Here's how the part is built. I have some questions about the finished solid (model axes, mm). A direction names the side the tool comes from. Round coordinates to 2 decimals unless told otherwise and drop trailing zeros. Order: outer loops, then holes, each group sorted by start corner. A loop starts at its lowest first (then second) coordinate and runs counter-clockwise, first axis right, second up. Notation, with made-up numbers: M 15,-14 L 20,-14 A14 cw 20,-8 Z; hole C 11.5,61.5 d6. An arc over 180 degrees is marked long. Write item = value, one per line. Start each with the question number.
Item 1: I'm going to push flat-ended pins straight in: P1, Ø10, axis at x = 41, z = 9.5, coming from the -Y side; P2, Ø10, axis at x = 25, z = 19.05, coming from the -Y side. Where does each tip first touch, or does it pass through?
Item 2: I want a section at C-C, the plane z = 0. List the corners of the cut face in (x, y) for me, plus the area to 3 significant figures.
Item 3: I want a section at D-D, the plane x = 6. List the corners of the cut face in (y, z) for me.
Item 4: Please list where these lines run through material, in increasing order: L1, parallel to Z at x = 41.5, y = 3.6; L2, parallel to Z at x = 25, y = 13.75; L3, parallel to Z at x = 41.5, y = 7.
Item 5: I want a section at B-B, the plane y = 4. List the corners of the cut face in (x, z) for me.
Item 6: For faces 1 (the face through (36, 15, -11)), 2 (the face through (44, 5.994, -7)), 3 (the face through (39.985, 14.113, 0.66)), which set-ups out of +Z, -Z, +X, -X, +Y, -Y let a thin tool reach every point of the face, with its end or its side?
Item 7: We'd pull the mould along X, two halves only. Please class faces 4 (the face through (1.528, 8.458, -23.551)), 5 (the face through (48.472, 8.458, -23.551)), 6 (the face through (27.52, 10.56, 17.12)): pulls with the +X half, pulls with the -X half, needs draft (parallel to the pull), parting line crosses it, or undercut.
Item 8: I want a section at A-A, the plane x = 25. List the corners of the cut face in (y, z) for me.
```python
from build123d import *

# Parameters (mm, degrees)
F1_DEPTH       = 50
F3_D           = 6.35
F3_CBORE_D     = 10.16
F3_CBORE_DEPTH = 5.9944
F5_DEPTH       = 50.001
F6_R           = 5.08
F7_R           = 15
F7_R_2         = 13
F8_DEPTH       = 1.8


with BuildPart() as f1:
    # F0 (on Right) → F1 (new body)
    with BuildSketch(Plane.YZ):
        Polygon((0, 25), (0, 0), (0, -25), (15, -25), (15, 25), align=None)
    extrude(amount=F1_DEPTH)

    # F3 (through all)
    with Locations(Plane.XZ):
        with Locations((25, 19.052559), (8.5, 9.526279), (41.5, 9.526279), (41.5, -9.526279), (25, -19.052559), (8.5, -9.526279)):
            CounterBoreHole(F3_D / 2, F3_CBORE_D / 2, F3_CBORE_DEPTH)

    # F4 (on face) → F5 (cut, through all)
    with BuildSketch(Plane.XY.offset(25)):
        Polygon((50, 0), (50, 3), (38, 0), align=None)
        Polygon((0, 0), (12, 0), (0, 3), align=None)
    extrude(amount=-F5_DEPTH, mode=Mode.SUBTRACT)

    # F6
    f6_edges = [f1.edges().sort_by_distance(p)[0] for p in [
        (50, 9, 25),
        (0, 9, 25),
        (0, 9, -25),
        (50, 9, -25),
    ]]
    fillet(f6_edges, radius=F6_R)

    # F7 (on face) → F8 (cut)
    with BuildSketch(Plane(origin=(0, 15, 0), x_dir=(-1, 0, 0), z_dir=(0, 1, 0))):
        with Locations((-25, 0)):
            Circle(F7_R)
        with Locations((-25, 0)):
            Circle(F7_R_2, mode=Mode.SUBTRACT)
    extrude(amount=-F8_DEPTH, mode=Mode.SUBTRACT)


solid = f1.part
```
Filled in:
q1.P1 = 0
q1.P2 = 5.99
q2.outline = M 0,3 L 12,0 L 38,0 L 50,3 L 50,15 L 40,15 L 40,13.2 L 38,13.2 L 38,15 L 12,15 L 12,13.2 L 10,13.2 L 10,15 L 0,15 Z
q2.area = 707 mm^2
q3.outline = M 1.5,-25 L 15,-25 L 15,-11.48 L 5.99,-11.48 L 5.99,-13.95 L 1.5,-13.95 Z; M 1.5,-5.1 L 5.99,-5.1 L 5.99,-7.57 L 15,-7.57 L 15,7.57 L 5.99,7.57 L 5.99,5.1 L 1.5,5.1 Z; M 1.5,13.95 L 5.99,13.95 L 5.99,11.48 L 15,11.48 L 15,25 L 1.5,25 Z
q4.L1 = -25 to -14.61, -4.45 to 4.45, 14.61 to 25
q4.L2 = -25 to -22.23, -15.88 to -15, -13 to 13, 15 to 15.88, 22.23 to 25
q4.L3 = -25 to -12.7, -6.35 to 6.35, 12.7 to 25
q5.outline = M 0,-19.92 A5.08 ccw 5.08,-25 L 44.92,-25 A5.08 ccw 50,-19.92 L 50,19.92 A5.08 ccw 44.92,25 L 5.08,25 A5.08 ccw 0,19.92 Z; hole C 8.5,-9.53 d10.16; hole C 8.5,9.53 d10.16; hole C 25,-19.05 d10.16; hole C 25,19.05 d10.16; hole C 41.5,-9.53 d10.16; hole C 41.5,9.53 d10.16
q6.face_1 = +Z, -Z, +X, -X, +Y
q6.face_2 = -Y
q6.face_3 = +Y
q7.face_4 = pulls with the -X half
q7.face_5 = pulls with the +X half
q7.face_6 = undercut
q8.outline = M 0,-25 L 15,-25 L 15,-22.23 L 5.99,-22.23 L 5.99,-24.13 L 0,-24.13 Z; M 0,-13.97 L 5.99,-13.97 L 5.99,-15.88 L 15,-15.88 L 15,-15 L 13.2,-15 L 13.2,-13 L 15,-13 L 15,13 L 13.2,13 L 13.2,15 L 15,15 L 15,15.88 L 5.99,15.88 L 5.99,13.97 L 0,13.97 Z; M 0,24.13 L 5.99,24.13 L 5.99,22.23 L 15,22.23 L 15,25 L 0,25 Z
